Work out the finished part from the listing and answer in its coordinate system (mm). A direction names the side the tool comes from. Round coordinates to 2 decimals unless told otherwise and drop trailing zeros. Loops run counter-clockwise (first coordinate to the right, second up) from the corner with the lowest first, then second, coordinate; pieces in that order, holes last.
```python
from build123d import *

# Parameters (mm, degrees)
BASE_FLANGE1_DEPTH            = 150
CUT_EXTRUDE1_REACH            = 154.095
SKETCH7_R                     = 2.5
EDGE_FLANGE1_STRIP_W          = 7
EDGE_FLANGE1_STRIP_H          = 1.25
EDGE_FLANGE1_STRIP_CUT_DEPTH  = 38
EDGE_FLANGE1_RELIEF_W         = 7.625
EDGE_FLANGE1_RELIEF_H         = 0.625
EDGE_FLANGE1_RELIEF_CUT_DEPTH = 1.25
EDGE_FLANGE1_DEPTH            = 38
EDGE_FLANGE2_STRIP_W          = 7
EDGE_FLANGE2_STRIP_H          = 1.25
EDGE_FLANGE2_STRIP_CUT_DEPTH  = 38
EDGE_FLANGE2_DEPTH            = 38
SKETCH14_W                    = 13
SKETCH14_H                    = 23.5
CUT_EXTRUDE2_DEPTH            = 1.25
EDGE_FLANGE3_STRIP_W          = 7
EDGE_FLANGE3_STRIP_H          = 1.25
EDGE_FLANGE3_STRIP_CUT_DEPTH  = 38
EDGE_FLANGE3_RELIEF_W         = 7.625
EDGE_FLANGE3_RELIEF_H         = 0.625
EDGE_FLANGE3_RELIEF_CUT_DEPTH = 1.25
EDGE_FLANGE3_DEPTH            = 38
EDGE_FLANGE4_STRIP_W          = 7
EDGE_FLANGE4_STRIP_H          = 1.25
EDGE_FLANGE4_STRIP_CUT_DEPTH  = 38
EDGE_FLANGE4_DEPTH            = 38
SKETCH21_W                    = 13
SKETCH21_H                    = 23.5
CUT_EXTRUDE3_DEPTH            = 1.25


# Sheet-metal steps are written as plain solids
with BuildPart() as part:
    # Sketch2 → Base-Flange1 (new body)
    with BuildSketch(Plane(origin=(0, 0, 0), x_dir=(1, 0, 0), z_dir=(0, 1, 0))):
        with BuildLine():
            Line((-10, -10), (-10, 9))
            ThreePointArc((-10, 9), (-9.707106781, 9.707106781), (-9, 10))
            Line((-9, 10), (9, 10))
            ThreePointArc((9, 10), (9.707106781, 9.707106781), (10, 9))
            Line((10, 9), (10, -10))
            Line((10, -10), (11.25, -10))
            Line((11.25, -10), (11.25, 9))
            ThreePointArc((11.25, 9), (10.590990258, 10.590990258), (9, 11.25))
            Line((9, 11.25), (-9, 11.25))
            ThreePointArc((-9, 11.25), (-10.590990258, 10.590990258), (-11.25, 9))
            Line((-11.25, 9), (-11.25, -10))
            Line((-11.25, -10), (-10, -10))
        make_face()
    extrude(amount=BASE_FLANGE1_DEPTH)

    # Cut-Extrude1: up to this face of the body (flat: up to its plane)
    cut_extrude1_end = Plane(part.part.faces().sort_by_distance((11.25, 75, 0.5))[0])
    # Sketch7 → Cut-Extrude1 (cut, up to the picked face)
    with BuildSketch(Plane.ZY.offset(11.25), mode=Mode.PRIVATE) as cut_extrude1_sk1:
        with Locations((-0.625, 12.5)):
            Circle(SKETCH7_R)
    cut_extrude1_tool1 = split(extrude(cut_extrude1_sk1.sketch, amount=-CUT_EXTRUDE1_REACH, mode=Mode.PRIVATE), bisect_by=cut_extrude1_end, keep=Keep.BOTH, mode=Mode.PRIVATE)
    # Sketch7 → Cut-Extrude1 (cut, up to the picked face)
    with BuildSketch(Plane.ZY.offset(11.25), mode=Mode.PRIVATE) as cut_extrude1_sk2:
        with Locations((-0.625, 137.5)):
            Circle(SKETCH7_R)
    cut_extrude1_tool2 = split(extrude(cut_extrude1_sk2.sketch, amount=-CUT_EXTRUDE1_REACH, mode=Mode.PRIVATE), bisect_by=cut_extrude1_end, keep=Keep.BOTH, mode=Mode.PRIVATE)
    add(cut_extrude1_tool1.solids().sort_by(Axis((-11.25, 12.5, -0.625), (1, 0, 0)))[0], mode=Mode.SUBTRACT)
    add(cut_extrude1_tool2.solids().sort_by(Axis((-11.25, 137.5, -0.625), (1, 0, 0)))[0], mode=Mode.SUBTRACT)

    # Edge-Flange1 strip (across the edge) → Edge-Flange1 strip cut (cut)
    with BuildSketch(Plane(origin=(11.25, 38, 10), x_dir=(0, 0, -1), z_dir=(0, -1, 0))):
        with Locations((-1.25, -0.625)):
            Rectangle(EDGE_FLANGE1_STRIP_W, EDGE_FLANGE1_STRIP_H)
    extrude(amount=EDGE_FLANGE1_STRIP_CUT_DEPTH, mode=Mode.SUBTRACT)

    # Edge-Flange1 relief (on the sheet) → Edge-Flange1 relief cut (cut)
    with BuildSketch(Plane(origin=(11.25, 38, 7.75), x_dir=(0, 0, -1), z_dir=(1, 0, 0))):
        with Locations((-3.1875, 0.3125)):
            Rectangle(EDGE_FLANGE1_RELIEF_W, EDGE_FLANGE1_RELIEF_H)
    extrude(amount=-EDGE_FLANGE1_RELIEF_CUT_DEPTH, mode=Mode.SUBTRACT)

    # Edge-Flange1 section (across the edge) → Edge-Flange1 (add)
    with BuildSketch(Plane(origin=(11.25, 38, 10), x_dir=(0, 0, -1), z_dir=(0, -1, 0))):
        with BuildLine():
            Line((0, 1), (0, 10.75))
            Line((0, 10.75), (1.25, 10.75))
            Line((1.25, 10.75), (1.25, 1))
            ThreePointArc((1.25, 1), (1.542893219, 0.292893219), (2.25, 0))
            Line((2.25, 0), (2.25, -1.25))
            ThreePointArc((2.25, -1.25), (0.659009742, -0.590990258), (0, 1))
        make_face()
    extrude(amount=EDGE_FLANGE1_DEPTH)

    # Edge-Flange2 strip (across the edge) → Edge-Flange2 strip cut (cut)
    with BuildSketch(Plane(origin=(22, 38, 8.75), x_dir=(-1, 0, 0), z_dir=(0, -1, 0))):
        with Locations((-1.25, -0.625)):
            Rectangle(EDGE_FLANGE2_STRIP_W, EDGE_FLANGE2_STRIP_H)
    extrude(amount=EDGE_FLANGE2_STRIP_CUT_DEPTH, mode=Mode.SUBTRACT)

    # Edge-Flange2 section (across the edge) → Edge-Flange2 (add)
    with BuildSketch(Plane(origin=(22, 38, 8.75), x_dir=(-1, 0, 0), z_dir=(0, -1, 0))):
        with BuildLine():
            Line((0, 1), (0, 15.75))
            Line((0, 15.75), (1.25, 15.75))
            Line((1.25, 15.75), (1.25, 1))
            ThreePointArc((1.25, 1), (1.542893219, 0.292893219), (2.25, 0))
            Line((2.25, 0), (2.25, -1.25))
            ThreePointArc((2.25, -1.25), (0.659009742, -0.590990258), (0, 1))
        make_face()
    extrude(amount=EDGE_FLANGE2_DEPTH)

    # Sketch14 → Cut-Extrude2 (cut)
    with BuildSketch(Plane(origin=(22, 0, 0), x_dir=(0, 0, -1), z_dir=(1, 0, 0))):
        with Locations((0.5, 17.75)):
            Rectangle(SKETCH14_W, SKETCH14_H)
    extrude(amount=-CUT_EXTRUDE2_DEPTH, mode=Mode.SUBTRACT)

    # Edge-Flange3 strip (across the edge) → Edge-Flange3 strip cut (cut)
    with BuildSketch(Plane(origin=(11.25, 150, 10), x_dir=(0, 0, -1), z_dir=(0, -1, 0))):
        with Locations((-1.25, -0.625)):
            Rectangle(EDGE_FLANGE3_STRIP_W, EDGE_FLANGE3_STRIP_H)
    extrude(amount=EDGE_FLANGE3_STRIP_CUT_DEPTH, mode=Mode.SUBTRACT)

    # Edge-Flange3 relief (on the sheet) → Edge-Flange3 relief cut (cut)
    with BuildSketch(Plane(origin=(11.25, 150, 7.75), x_dir=(0, 0, -1), z_dir=(1, 0, 0))):
        with Locations((-3.1875, -38.3125)):
            Rectangle(EDGE_FLANGE3_RELIEF_W, EDGE_FLANGE3_RELIEF_H)
    extrude(amount=-EDGE_FLANGE3_RELIEF_CUT_DEPTH, mode=Mode.SUBTRACT)

    # Edge-Flange3 section (across the edge) → Edge-Flange3 (add)
    with BuildSketch(Plane(origin=(11.25, 150, 10), x_dir=(0, 0, -1), z_dir=(0, -1, 0))):
        with BuildLine():
            Line((0, 1), (0, 10.75))
            Line((0, 10.75), (1.25, 10.75))
            Line((1.25, 10.75), (1.25, 1))
            ThreePointArc((1.25, 1), (1.542893219, 0.292893219), (2.25, 0))
            Line((2.25, 0), (2.25, -1.25))
            ThreePointArc((2.25, -1.25), (0.659009742, -0.590990258), (0, 1))
        make_face()
    extrude(amount=EDGE_FLANGE3_DEPTH)

    # Edge-Flange4 strip (across the edge) → Edge-Flange4 strip cut (cut)
    with BuildSketch(Plane(origin=(22, 150, 8.75), x_dir=(-1, 0, 0), z_dir=(0, -1, 0))):
        with Locations((-1.25, -0.625)):
            Rectangle(EDGE_FLANGE4_STRIP_W, EDGE_FLANGE4_STRIP_H)
    extrude(amount=EDGE_FLANGE4_STRIP_CUT_DEPTH, mode=Mode.SUBTRACT)

    # Edge-Flange4 section (across the edge) → Edge-Flange4 (add)
    with BuildSketch(Plane(origin=(22, 150, 8.75), x_dir=(-1, 0, 0), z_dir=(0, -1, 0))):
        with BuildLine():
            Line((0, 1), (0, 15.75))
            Line((0, 15.75), (1.25, 15.75))
            Line((1.25, 15.75), (1.25, 1))
            ThreePointArc((1.25, 1), (1.542893219, 0.292893219), (2.25, 0))
            Line((2.25, 0), (2.25, -1.25))
            ThreePointArc((2.25, -1.25), (0.659009742, -0.590990258), (0, 1))
        make_face()
    extrude(amount=EDGE_FLANGE4_DEPTH)

    # Sketch21 → Cut-Extrude3 (cut)
    with BuildSketch(Plane(origin=(22, 0, 0), x_dir=(0, 0, -1), z_dir=(1, 0, 0))):
        with Locations((0.5, 132.25)):
            Rectangle(SKETCH21_W, SKETCH21_H)
    extrude(amount=-CUT_EXTRUDE3_DEPTH, mode=Mode.SUBTRACT)


solid = part.part
```
1. Find section A-A (y = 137.5). Write down the section's boundary in (x, z) (3 decimals).
Answer key:
outline: (-11.25, -9) arc R2.25 ccw to (-9, -11.25) - (9, -11.25) arc R2.25 ccw to (11.25, -9) - (11.25, -3.125) - (10, -3.125) - (10, -9) arc R1 cw to (9, -10) - (-9, -10) arc R1 cw to (-10, -9) - (-10, -3.125) - (-11.25, -3.125) - close; (-11.25, 1.875) - (-10, 1.875) - (-10, 10) - (-11.25, 10) - close; (10, 1.875) - (11.25, 1.875) - (11.25, 7.75) arc R1 cw to (12.25, 8.75) - (19.75, 8.75) arc R1 cw to (20.75, 7.75) - (20.75, 6) - (22, 6) - (22, 7.75) arc R2.25 ccw to (19.75, 10) - (12.25, 10) arc R2.25 ccw to (10, 7.75) - close
2. Given pin 1 (1 mm diameter, centred on y = 83, z = 0.5, fed in from +X); pin 2 (4.5 mm diameter, centred on y = 12.5, z = -0.625, fed in from -X); pin 3 (0.6 mm diameter, centred on x = 21.5, y = 116.5, fed in from -Z); pin 4 (14.5 mm diameter, centred on x = 1, y = 112, fed in from +Z), each flat-ended and moving along its own axis, determine where each tip first touches the part or whether it passes through.
Answer key:
pin 1: stops at x = 11.25
pin 2: passes through
pin 3: stops at z = -7
pin 4: stops at z = -10
3. Find section D-D (z = -1.5). Give the number of separate pieces and of enclosed holes in the cut face, then the cut area to 3 significant figures.
Answer key:
separate pieces: 10
enclosed holes: 0
area: 388 mm2
4. Determine the mould class of faces 1 (the face through (22, 23, 7)), 2 (the face through (21, 38, 4)), 3 (the face through (20.75, 23, 7)) for opening direction X: +X half, -X half, draft (parallel to the pull), parting line (faces both ways), or undercut.
Answer key:
face 1: +X half
face 2: draft
face 3: undercut
5. Find section C-C (x = 7.5). Write down the section's boundary in (y, z).
Answer key:
outline: (0, -11.25) - (150, -11.25) - (150, -10) - (0, -10) - close
6. Find section B-B (y = 101.5). Write down the section's boundary in (x, z), then the cut area to 3 significant figures.
Answer key:
outline: (-11.25, -9) arc R2.25 ccw to (-9, -11.25) - (9, -11.25) arc R2.25 ccw to (11.25, -9) - (11.25, 10) - (10, 10) - (10, -9) arc R1 cw to (9, -10) - (-9, -10) arc R1 cw to (-10, -9) - (-10, 10) - (-11.25, 10) - close
area: 76.4 mm2
7. Consider probe 1 along X at (y, z) = (32.5, -5); probe 2 along X at (y, z) = (118, 8); probe 3 along X at (y, z) = (127, 4). Determine where each line is inside the solid, lowest interval first.
Answer key:
probe 1: x = -11.25 to -10, 10 to 11.25, 20.75 to 22
probe 2: x = -11.25 to -10, 10.01 to 11.28, 20.72 to 21.99
probe 3: x = -11.25 to -10, 10 to 11.25
8. Which of the six approach directions +Z, -Z, +X, -X, +Y, -Y give full straight-line access (tool end or side, diameter ignored) to faces 4 (the face through (-10.63, 10.06, -1.17)), 5 (the face through (16, 131, 8.75)), 6 (the face through (0, 74, -10))?
Answer key:
face 4: +X, -X
face 5: -Z, +Y, -Y
face 6: +Z, +Y, -Y
